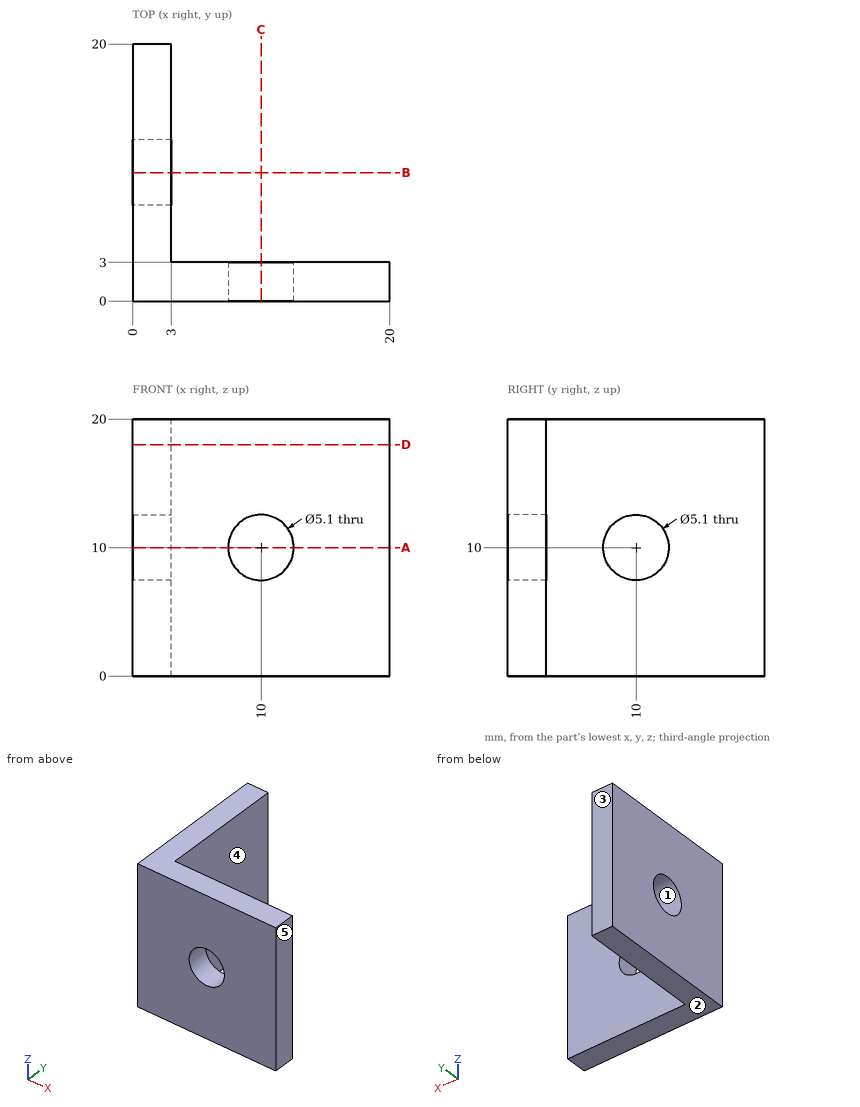
Here's the drawing with two shaded views (mm, measured from the low corner). I have some questions. A direction names the side the tool comes from. Coordinates: 2 decimals unless noted, no trailing zeros. Write each loop counter-clockwise with the first axis right and the second up, starting at its lowest first coordinate (ties: lowest second). Pieces come first, ordered by that corner, then holes. Notation, with made-up numbers: (42, -14) -> (94, -14) arc R9 ccw to (94, -6) -> close; hole circle Ø1 at (-32.75, -1). An arc over 180 degrees is marked (long way). Answer as CSV lines item,"result".
1) If I drill on line 1 (Y direction, x = 0.9, z = 10); line 2 (Y direction, x = 7.5, z = 11.5), over which ranges is the centre line in solid material (lowest first)? Write a range as from..to.
Check result:
line 1,"0..7.45, 12.55..20"
line 2,"0..3"
2) On a 3-axis mill with a long thin cutter (end or side, diameter ignored), from which of +Z, -Z, +X, -X, +Y, -Y can I reach the whole of each face in a straight line? I mean the marked faces 4 and 5. Say none if no direction works.
Check result:
face 4,"+Z, -Z, +X, +Y"
face 5,"+Z, -Z, +X, +Y, -Y"
3) If we section it at A-A on z = 10: Please give me the cut outline in (x, y).
Check result:
outline,"(0, 0) -> (7.45, 0) -> (7.45, 3) -> (3, 3) -> (3, 7.45) -> (0, 7.45) -> close; (0, 12.55) -> (3, 12.55) -> (3, 20) -> (0, 20) -> close; (12.55, 0) -> (20, 0) -> (20, 3) -> (12.55, 3) -> close"
4) If we mould it in two halves opening along Y, with no side actions, what happens to the marked faces 1, 2 and 3? For each: +Y half, -Y half, draft (parallel to the pull), parting line (faces both ways), or undercut.
Check result:
face 1,"undercut"
face 2,"draft"
face 3,"+Y half"
5) If we section it at D-D on z = 18: Please give me the cut outline in (x, y), then the cut area to 3 significant figures.
Check result:
outline,"(0, 0) -> (20, 0) -> (20, 3) -> (3, 3) -> (3, 20) -> (0, 20) -> close"
area,"111 mm²"
6) Will these pins go through, and if not, where does the flat tip stop? P1, Ø5, axis at x = 17.5, z = 5.5, coming from the +Y side; P2, Ø8, axis at y = 10, z = 10, coming from the +X side.
Check result:
P1,"y = 3"
P2,"x = 3"
7) If we section it at B-B on y = 10: Please give me the cut outline in (x, z), then the cut area to 3 significant figures.
Check result:
outline,"(0, 0) -> (3, 0) -> (3, 7.45) -> (0, 7.45) -> close; (0, 12.55) -> (3, 12.55) -> (3, 20) -> (0, 20) -> close"
area,"44.7 mm²"
